The listing builds one solid part. Answer for the finished solid, in the listing's coordinates (mm). Face numbers are marked on the shaded views. A direction names the side the tool comes from. Coordinates: 2 decimals unless noted, no trailing zeros. Order: outer loops, then holes, each group sorted by start corner. A loop starts at its lowest first (then second) coordinate and runs counter-clockwise, first axis right, second up. Notation, with made-up numbers: (51, 38.5) -> (97, 38.5) arc R28 cw to (97, 72.5) -> close; hole circle Ø7 at (81.5, 49). An arc over 180 degrees is marked (long way). Write each question's results on one line, items separated by ' | '. Start each with the question number.
(1) Given pin 1 (4 mm diameter, centred on x = 6, z = -41.5, fed in from +Y) (1 decimal); pin 2 (3 mm diameter, centred on x = 35.5, y = 3.5, fed in from -Z), each flat-ended and moving along its own axis, determine where each tip first touches the part or whether it passes through.
(2) Determine the mould class of the marked faces 3, 4 and 5 for opening direction Z: +Z half, -Z half, draft (parallel to the pull), parting line (faces both ways), or undercut.
(3) A tool of negligible diameter and unlimited length cuts with its end or side. For the marked faces 1 and 2, from which of +Z, -Z, +X, -X, +Y, -Y can it reach the whole face along a straight path? Write none if from no direction.
(4) The part is cut by section D-D, the plane z = -20. Give the vertices of the cut face in (x, y).
(5) The part is cut by section C-C, the plane x = 19. Give the vertices of the cut face in (y, z).
(6) The part is cut by section B-B, the plane y = 8.25. Give the vertices of the cut face in (x, z).
(7) Straight lines are drawn through the part: L1, parallel to Z at x = 0, y = 9; L2, parallel to X at y = 3.5, z = -49; L3, parallel to Z at x = 36.5, y = 10.5. For each, find the intervals that lie inside material, in ascending order.
(8) The part is cut by section A-A, the plane z = -49. Give the vertices of the cut face in (x, y), then the cut area to 3 significant figures.
```python
from build123d import *

# Parameters (mm, degrees)
SKETCH1_R           = 2.7
BOSS_EXTRUDE1_DEPTH = 13
FILLET1_R           = 0.8


with BuildPart() as part:
    # Sketch1 → Boss-Extrude1 (new body)
    with BuildSketch(Plane(origin=(0, 0, 0), x_dir=(1, 0, 0), z_dir=(0, 1, 0))):
        with BuildLine():
            Line((51.921017872, 32.018867925), (0, 53))
            ThreePointArc((0, 53), (-4, 49), (0, 45))
            ThreePointArc((0, 45), (40.783850417, 19.017821778), (34.47199994, -28.925442436))
            ThreePointArc((34.47199994, -28.925442436), (34.965027274, -34.560770647), (40.600355485, -34.067743313))
            Line((40.600355485, -34.067743313), (37.536177713, -31.496592875))
            ThreePointArc((37.536177713, -31.496592875), (48.870327604, -3.562454189), (41.707047143, 25.720074234))
            Line((41.707047143, 25.720074234), (51.921017872, 32.018867925))
        make_face()
        with Locations((0, 49)):
            Circle(SKETCH1_R, mode=Mode.SUBTRACT)
    extrude(amount=BOSS_EXTRUDE1_DEPTH)

    # Fillet1
    fillet1_edges = [part.edges().sort_by_distance(p)[0] for p in [
        (51.921017872, 6.5, -32.018867925),
        (41.707047143, 6.5, -25.720074234),
        (37.536177713, 6.5, 31.496592875),
        (40.600355485, 6.5, 34.067743313),
        (0, 6.5, -53),
    ]]
    fillet(fillet1_edges, radius=FILLET1_R)


solid = part.part
```
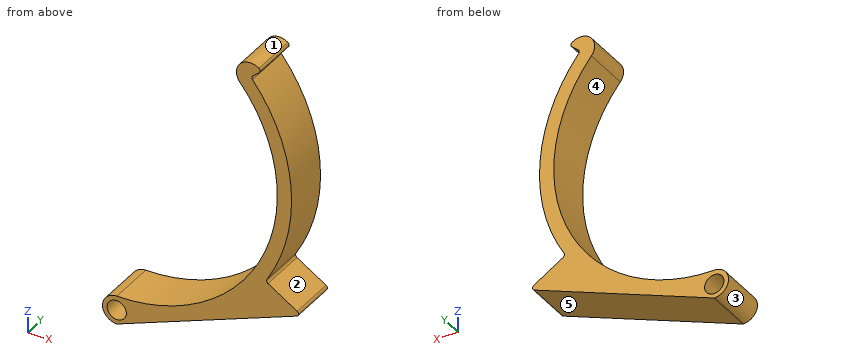
Established:
1) pin 1: passes through | pin 2: stops at z = -39.26
2) face 3: parting line | face 4: undercut | face 5: -Z half
3) face 1: +Y, -Y | face 2: +X, +Y, -Y
4) outline: (40.31, 0) -> (44.73, 0) -> (44.73, 13) -> (40.31, 13) -> close
5) outline: (0, -45.32) -> (13, -45.32) -> (13, -40.79) -> (0, -40.79) -> close
6) outline: (-0.18, -53) arc R0.8 ccw to (0.15, -52.94) -> (50.45, -32.61) arc R0.8 ccw to (50.57, -31.19) -> (42.38, -26.14) arc R0.8 cw to (42.11, -25.05) arc R49 ccw to (38.04, 30.89) arc R0.8 cw to (38.14, 32.01) -> (39.91, 33.49) arc R0.8 ccw to (39.86, 34.75) arc R4 ccw to (34.47, 28.93) arc R45 cw to (0, -45) arc R4 ccw to start; hole circle Ø5.4 at (0, -49)
7) L1: z = -52.98 to -51.7, -46.3 to -45 | L2: x = -4 to -2.7, 2.7 to 9.9 | L3: z = -38.25 to -26.32, 26.32 to 35.36
8) outline: (-4, 0) -> (-2.7, 0) -> (-2.7, 13) -> (-4, 13) -> close; (2.7, 0) -> (9.9, 0) -> (9.9, 13) -> (2.7, 13) -> close | area: 110 mm^2
